from build123d import *

# Parameters (mm, degrees)
BOSS_EXTRUDE1_DEPTH            = 6
CBORE_FOR_M4_SHCS1_D           = 4.3
CBORE_FOR_M4_SHCS1_CBORE_D     = 8
CBORE_FOR_M4_SHCS1_CBORE_DEPTH = 4


with BuildPart() as part:
    # Sketch1 → Boss-Extrude1 (new, symmetric)
    with BuildSketch(Plane.XY):
        with BuildLine():
            Line((20, 0), (-20, 0))
            Line((-20, 0), (-20, 10))
            Line((-20, 10), (-4.736180555, 10))
            ThreePointArc((-4.736180555, 10), (0, 5.7375), (4.736180555, 10))
            Line((4.736180555, 10), (20, 10))
            Line((20, 10), (20, 0))
        make_face()
    extrude(amount=BOSS_EXTRUDE1_DEPTH, both=True)

    # CBORE for M4 SHCS1 (through all)
    with Locations(Plane.XZ):
        with Locations((-11.9365, 0), (11.9365, 0)):
            CounterBoreHole(CBORE_FOR_M4_SHCS1_D / 2, CBORE_FOR_M4_SHCS1_CBORE_D / 2, CBORE_FOR_M4_SHCS1_CBORE_DEPTH)


solid = part.part
The listing builds one solid part. Answer for the finished solid, in the listing's coordinates (mm). A direction names the side the tool comes from. Give positions to 0.01 mm unless a question says otherwise; leave off trailing zeros. Loops run counter-clockwise (first coordinate to the right, second up) from the corner with the lowest first, then second, coordinate; pieces in that order, holes last.
Item 1: Determine the mould class of faces 3 (the flat face through (14, 4, -2)), 4 (the flat face through (20, 5, 0)), 5 (the flat face through (0, 5, 6)) for opening direction Z: +Z half, -Z half, draft (parallel to the pull), parting line (faces both ways), or undercut.
Derived:
face 3: undercut
face 4: draft
face 5: +Z half
Item 2: A tool of negligible diameter and unlimited length cuts with its end or side. For faces 1 (the cylindrical face through (8.76, 1.97, -2.43)), 2 (the cylindrical face through (-9.79, 7.04, 0.09)), from which of +Z, -Z, +X, -X, +Y, -Y can it reach the whole face along a straight path? Write none if from no direction.
Derived:
face 1: -Y
face 2: +Y, -Y
Item 3: A cutting plane is placed at C-C (x = -13). Give the vertices of the cut face in (y, z), then the cut area to 3 significant figures.
Derived:
outline: (0, -6) - (10, -6) - (10, -1.87) - (4, -1.87) - (4, -3.86) - (0, -3.86) - close; (0, 3.86) - (4, 3.86) - (4, 1.87) - (10, 1.87) - (10, 6) - (0, 6) - close
area: 66.7 mm2
Item 4: Find the intervals of material crossed by line 1 along X through (y, z) = (9.25, -1.25); line 2 along X through (y, z) = (3, -0.5); line 3 along Y through (x, z) = (-12, 2.25), in increasing order.
Derived:
line 1: x = -20 to -13.69, -10.19 to -4.6, 4.6 to 10.19, 13.69 to 20
line 2: x = -20 to -15.91, -7.97 to 7.97, 15.91 to 20
line 3: y = 4 to 10
Item 5: A cutting plane is placed at B-B (z = 0). Give the vertices of the cut face in (x, y) (1 decimal), then the cut area to 3 significant figures.
Derived:
outline: (-20, 0) - (-15.9, 0) - (-15.9, 4) - (-14.1, 4) - (-14.1, 10) - (-20, 10) - close; (-9.8, 4) - (-7.9, 4) - (-7.9, 0) - (7.9, 0) - (7.9, 4) - (9.8, 4) - (9.8, 10) - (4.7, 10) arc R4.8 cw to (-4.7, 10) - (-9.8, 10) - close; (14.1, 4) - (15.9, 4) - (15.9, 0) - (20, 0) - (20, 10) - (14.1, 10) - close
area: 254 mm2
Item 6: This flat-tipped pin is pushed along its axis until it touches: pin 1 Ø4 at (x, z) = (-10.5, 1) entering from -Y. Where does it stop, or does it pass through?
Derived:
pin 1: stops at y = 4
Item 7: A cutting plane is placed at D-D (y = 3.5). Give the vertices of the cut face in (x, z).
Derived:
outline: (-20, -6) - (20, -6) - (20, 6) - (-20, 6) - close; hole circle Ø8 at (-11.94, 0); hole circle Ø8 at (11.94, 0)
Item 8: A cutting plane is placed at A-A (y = 8). Give the vertices of the cut face in (x, z).
Derived:
outline: (-20, -6) - (-4.05, -6) - (-4.05, 6) - (-20, 6) - close; (4.05, -6) - (20, -6) - (20, 6) - (4.05, 6) - close; hole circle Ø4.3 at (-11.94, 0); hole circle Ø4.3 at (11.94, 0)
